Autodesk Inventor part; units mm, degrees
ref_plane "YZ Plane" through (0, 0, 0) normal (1, 0, 0) x (0, 1, 0)
ref_plane "XZ Plane" through (0, 0, 0) normal (0, 1, 0) x (-1, 0, 0)
ref_plane "XY Plane" through (0, 0, 0) normal (0, 0, 1) x (1, 0, 0)
sketch "Эскиз1" plane through (0, 0, 0) normal (0, 1, 0) x (-1, 0, 0)
  circle A0 centre (0, 0) radius 2.75
  circle A1 centre (0, 0) radius 5.5
  dimension "d0" = 5.5
  dimension "d1" = 11
extrude "Выдавливание1" add sketch "Эскиз1" along normal blind 6.6
fillet "Сопряжение1" radius 0.8 2 edges at (5.5, 6.6, 0) (5.5, 0, 0)
chamfer "Фаска1" distance 0.6 angle 45 2 edges at (2.75, 6.6, 0) (2.75, 0, 0)
properties part number "prostavka_6,6"
Design review of the part built by this model. Coordinates are the model's own, in mm. Round coordinates to 2 decimals unless told otherwise and drop trailing zeros. Write each loop counter-clockwise with the first axis right and the second up, starting at its lowest first coordinate (ties: lowest second). Pieces come first, ordered by that corner, then holes.
Item 1: Clearance check with a flat-ended pin moving along its axis: pin 1 Ø2 at (y, z) = (4.5, 2) entering from +X. State where the tip first meets the part, or that it passes through.
Item 2: We need section B-B on z = 0. Write out the cut boundary in (x, y), and give its area (3 significant figures).
Item 3: For probe 1 along Z at (x, y) = (0, 3.4); probe 2 along Z at (x, y) = (1.5, 1.5); probe 3 along X at (y, z) = (5.5, -0.5), list the stretches that pass through material, from the lowest coordinate up.
Item 4: We need section C-C on y = 1. Write out the cut boundary in (x, z).
Item 5: We need section D-D on y = 6.25. Write out the cut boundary in (x, z).
Item 6: The part is to be moulded in two halves that separate along X. For faces 1 (the cylindrical face through (1.19, 3.26, 5.37)), 2 (the cylindrical face through (0.596, 3.262, 2.685)), 3 (the flat face through (-3, 6.6, -2)), say which applies: +X half, -X half, draft (parallel to the pull), parting line (faces both ways), or undercut.
Item 7: We need section A-A on x = 0. Write out the cut boundary in (y, z), and give its area (3 significant figures).
Returned:
1. pin 1: stops at x = 5.41
2. outline: (-5.5, 0.8) arc R0.8 ccw to (-4.7, 0) - (-3.35, 0) - (-2.75, 0.6) - (-2.75, 6) - (-3.35, 6.6) - (-4.7, 6.6) arc R0.8 ccw to (-5.5, 5.8) - close; (2.75, 0.6) - (3.35, 0) - (4.7, 0) arc R0.8 ccw to (5.5, 0.8) - (5.5, 5.8) arc R0.8 ccw to (4.7, 6.6) - (3.35, 6.6) - (2.75, 6) - close
2. area: 35.0 mm2
3. probe 1: z = -5.5 to -2.75, 2.75 to 5.5
3. probe 2: z = -5.29 to -2.3, 2.3 to 5.29
3. probe 3: x = -5.48 to -2.7, 2.7 to 5.48
4. outline: circle Ø11 at (0, 0); hole circle Ø5.5 at (0, 0)
5. outline: circle Ø10.72 at (0, 0); hole circle Ø6 at (0, 0)
6. face 1: parting line
6. face 2: undercut
6. face 3: draft
7. outline: (0, -4.7) arc R0.8 ccw to (0.8, -5.5) - (5.8, -5.5) arc R0.8 ccw to (6.6, -4.7) - (6.6, -3.35) - (6, -2.75) - (0.6, -2.75) - (0, -3.35) - close; (0, 3.35) - (0.6, 2.75) - (6, 2.75) - (6.6, 3.35) - (6.6, 4.7) arc R0.8 ccw to (5.8, 5.5) - (0.8, 5.5) arc R0.8 ccw to (0, 4.7) - close
7. area: 35.0 mm2
